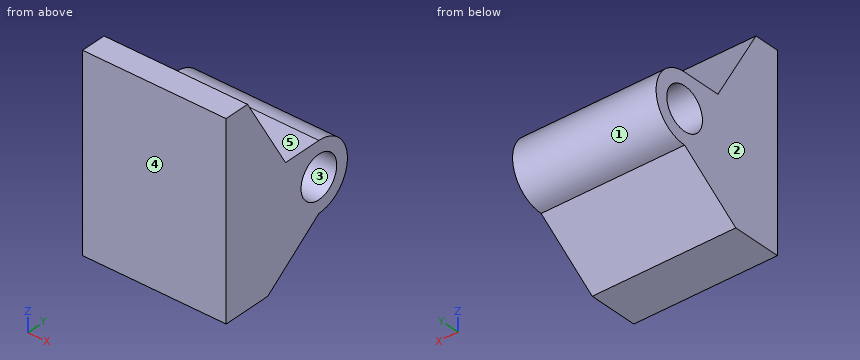
from build123d import *

# Parameters (mm, degrees)
EXTRUDE_START   = 0.633192
SKETCH_1_R      = 15
EXTRUDE_3_DEPTH = 102


with BuildPart() as part:
    # Эскиз1 → Бобышка-Вытянуть3 (new body)
    with BuildSketch(Plane(origin=(0, 0, 0), x_dir=(0, 0, -1), z_dir=(1, 0, 0)).offset(EXTRUDE_START)):
        with BuildLine():
            Line((0, 0), (0, 35))
            Line((0, 35), (-32, 78))
            ThreePointArc((-32, 78), (-56, 102), (-80, 78))
            Line((-80, 78), (-80, 50))
            Line((-80, 50), (-135, 18))
            Line((-135, 18), (-135, 0))
            Line((-135, 0), (0, 0))
        make_face()
        with Locations((-56, 78)):
            Circle(SKETCH_1_R, mode=Mode.SUBTRACT)
    extrude(amount=EXTRUDE_3_DEPTH)


solid = part.part
Read the model definition and answer for the solid it produces. Units are mm, in the model's axes. Face numbers are marked on the shaded views. A direction names the side the tool comes from. Round coordinates to 2 decimals unless told otherwise and drop trailing zeros. Write each loop counter-clockwise with the first axis right and the second up, starting at its lowest first coordinate (ties: lowest second). Pieces come first, ordered by that corner, then holes.
Q1. Straight lines are drawn through the part: line 1 (Z direction, x = 77.5, y = 78.5); line 2 (Y direction, x = 80.5, z = 56); line 3 (Z direction, x = 69, y = 64.5). For each, find the intervals that lie inside material, in ascending order.
Values:
line 1: z = 32.01 to 41.01, 70.99 to 79.99
line 2: y = 0 to 63, 93 to 102
line 3: z = 21.95 to 49.46, 62.54 to 80
Q2. A tool of negligible diameter and unlimited length cuts with its end or side. For the marked faces 4 and 5, from which of +Z, -Z, +X, -X, +Y, -Y can it reach the whole face along a straight path? Write none if from no direction.
Values:
face 4: +Z, -Z, +X, -X, -Y
face 5: +Z, +X, -X, +Y
Q3. Find section A-A on x = 33. Determine the outline of the cut face in (y, z), and give its area (3 significant figures).
Values:
outline: (0, 0) - (35, 0) - (78, 32) arc R24 ccw to (78, 80) - (50, 80) - (18, 135) - (0, 135) - close; hole circle Ø30 at (78, 56)
area: 7,620 mm2
Q4. Flat-ended cylindrical pins translate along their axes: P1, Ø12, axis at x = 54, z = 86.5, coming from the +Y side; P2, Ø14, axis at x = 36, y = 66, coming from the +Z side; P3, Ø4, axis at x = 17.5, y = 70, coming from the -Z side. Find the tip coordinate at first contact, or state that the pin passes through.
Values:
P1: stops at y = 49.71
P2: stops at z = 80
P3: stops at z = 24.56
Q5. Find section C-C on y = 84. Determine the outline of the cut face in (x, z), and give its area (3 significant figures).
Values:
outline: (0.63, 32.76) - (102.63, 32.76) - (102.63, 42.25) - (0.63, 42.25) - close; (0.63, 69.75) - (102.63, 69.75) - (102.63, 79.24) - (0.63, 79.24) - close
area: 1,940 mm2
Q6. Find section B-B on z = 56. Determine the outline of the cut face in (x, y), and give its area (3 significant figures).
Values:
outline: (0.63, 0) - (102.63, 0) - (102.63, 63) - (0.63, 63) - close; (0.63, 93) - (102.63, 93) - (102.63, 102) - (0.63, 102) - close
area: 7,340 mm2
Q7. The mould has two halves that part along Y. Classify the marked faces 1, 2 and 3: released by +Y, released by -Y, zero draft, split by the parting line, or undercut.
Values:
face 1: released by +Y
face 2: zero draft
face 3: undercut
Q8. Find section D-D on y = 43.5. Determine the outline of the cut face in (x, z), and give its area (3 significant figures).
Values:
outline: (0.63, 6.33) - (102.63, 6.33) - (102.63, 91.17) - (0.63, 91.17) - close
area: 8,650 mm2
